The listing builds one solid part. Answer for the finished solid, in the listing's coordinates (mm). Coordinates: 2 decimals unless noted, no trailing zeros. Order: outer loops, then holes, each group sorted by start corner. A loop starts at its lowest first (then second) coordinate and runs counter-clockwise, first axis right, second up. Notation, with made-up numbers: (25, 13.5) -> (83, 13.5) arc R24 ccw to (83, 44.5) -> close; hole circle Ø10 at (-33.75, 76.5). An arc over 180 degrees is marked (long way). One line per question, with ' | ' between items.
from build123d import *

# Parameters (mm, degrees)
BASE_DEPTH                = 3
ESQUISSE3_R               = 2
ESQUISSE3_W               = 65
ESQUISSE3_H               = 30
ENL_V_MAT_EXTRU_1_DEPTH   = 4
CONG_1_R                  = 3
ESQUISSE6_R               = 2
ESQUISSE6_R_2             = 10.5
PER_AGE_POUR_BILLES_DEPTH = 3
PER_AGE_POUR_PROFIL_REACH = 5
ESQUISSE8_R               = 3
ESQUISSE10_R              = 2
ENL_V_MAT_EXTRU_3_DEPTH   = 4
ESQUISSE12_R              = 1.625
ENL_V_MAT_EXTRU_4_DEPTH   = 4
ESQUISSE13_R              = 1.625
ENL_V_MAT_EXTRU_5_DEPTH   = 4


with BuildPart() as part:
    # Esquisse1 → Base (new body)
    with BuildSketch(Plane.XY):
        Polygon((0, 0), (-150, 0), (-174.748737342, 24.748737342), (-174.748737342, 274.748737342), (-150, 299.497474683), (0, 299.497474683), (24.748737342, 274.748737342), (24.748737342, 24.748737342), align=None)
    extrude(amount=BASE_DEPTH)

    # Esquisse3 → Enlèv. mat.-Extru.1 (cut, through all)
    with BuildSketch(Plane(origin=(0, 0, 0), x_dir=(-1, 0, 0), z_dir=(0, 0, -1))):
        with Locations((40, 45)):
            Circle(ESQUISSE3_R)
        with Locations((110, 45)):
            Circle(ESQUISSE3_R)
        with Locations((110, 254.497474683)):
            Circle(ESQUISSE3_R)
        with Locations((40, 254.497474683)):
            Circle(ESQUISSE3_R)
        Polygon((117, 0), (117, 20), (93, 20), (93, 45.5), (57, 45.5), (57, 20), (33, 20), (33, 0), align=None)
        Polygon((33, 299.497474683), (117, 299.497474683), (117, 279.497474683), (93, 279.497474683), (93, 253.997474683), (57, 253.997474683), (57, 279.497474683), (33, 279.497474683), align=None)
        with Locations((75, 229.497474683)):
            Rectangle(ESQUISSE3_W, ESQUISSE3_H)
        with Locations((75, 70)):
            Rectangle(ESQUISSE3_W, ESQUISSE3_H)
    extrude(amount=-ENL_V_MAT_EXTRU_1_DEPTH, mode=Mode.SUBTRACT)

    # Congé1
    cong_1_edges = [part.edges().sort_by_distance(p)[0] for p in [
        (0, 0, 1.5),
        (-150, 0, 1.5),
        (-174.748737342, 24.748737342, 1.5),
        (-174.748737342, 274.748737342, 1.5),
        (-150, 299.497474683, 1.5),
        (0, 299.497474683, 1.5),
        (24.748737342, 274.748737342, 1.5),
        (24.748737342, 24.748737342, 1.5),
        (-33, 279.497474683, 1.5),
        (-33, 299.497474683, 1.5),
        (-117, 299.497474683, 1.5),
        (-117, 279.497474683, 1.5),
        (-93, 279.497474683, 1.5),
        (-93, 253.997474683, 1.5),
        (-57, 253.997474683, 1.5),
        (-57, 279.497474683, 1.5),
        (-117, 0, 1.5),
        (-33, 0, 1.5),
        (-33, 20, 1.5),
        (-57, 20, 1.5),
        (-57, 45.5, 1.5),
        (-93, 45.5, 1.5),
        (-93, 20, 1.5),
        (-117, 20, 1.5),
    ]]
    fillet(cong_1_edges, radius=CONG_1_R)

    # Esquisse6 → Perçage pour billes (cut)
    with BuildSketch(Plane.XY.offset(3)):
        with Locations((-152, 55)):
            Circle(ESQUISSE6_R)
        with Locations((-152, 85)):
            Circle(ESQUISSE6_R)
        with Locations((-152, 70)):
            Circle(ESQUISSE6_R_2)
        with Locations((-5.251262658, 40)):
            Circle(ESQUISSE6_R_2)
        with Locations((-20.251262658, 40)):
            Circle(ESQUISSE6_R)
        with Locations((9.748737342, 40)):
            Circle(ESQUISSE6_R)
    per_age_pour_billes = extrude(amount=-PER_AGE_POUR_BILLES_DEPTH, mode=Mode.SUBTRACT)

    # Esquisse8 → Perçage pour profilé (cut, up to next)
    with BuildSketch(Plane.XY.offset(3), mode=Mode.PRIVATE) as per_age_pour_profil_sk1:
        with Locations((-133, 16)):
            Circle(ESQUISSE8_R)
    per_age_pour_profil_tool1 = extrude(per_age_pour_profil_sk1.sketch, amount=-PER_AGE_POUR_PROFIL_REACH, mode=Mode.PRIVATE) & part.part
    add(per_age_pour_profil_tool1.solids().sort_by_distance((-133, 16, 3))[0], mode=Mode.SUBTRACT)
    # Esquisse8 → Perçage pour profilé (cut, up to next)
    with BuildSketch(Plane.XY.offset(3), mode=Mode.PRIVATE) as per_age_pour_profil_sk2:
        with Locations((-133, 283.497474683)):
            Circle(ESQUISSE8_R)
    per_age_pour_profil_tool2 = extrude(per_age_pour_profil_sk2.sketch, amount=-PER_AGE_POUR_PROFIL_REACH, mode=Mode.PRIVATE) & part.part
    add(per_age_pour_profil_tool2.solids().sort_by_distance((-133, 283.497475, 3))[0], mode=Mode.SUBTRACT)
    # Esquisse8 → Perçage pour profilé (cut, up to next)
    with BuildSketch(Plane.XY.offset(3), mode=Mode.PRIVATE) as per_age_pour_profil_sk3:
        with Locations((-17, 283.497474683)):
            Circle(ESQUISSE8_R)
    per_age_pour_profil_tool3 = extrude(per_age_pour_profil_sk3.sketch, amount=-PER_AGE_POUR_PROFIL_REACH, mode=Mode.PRIVATE) & part.part
    add(per_age_pour_profil_tool3.solids().sort_by_distance((-17, 283.497475, 3))[0], mode=Mode.SUBTRACT)
    # Esquisse8 → Perçage pour profilé (cut, up to next)
    with BuildSketch(Plane.XY.offset(3), mode=Mode.PRIVATE) as per_age_pour_profil_sk4:
        with Locations((-17, 16)):
            Circle(ESQUISSE8_R)
    per_age_pour_profil_tool4 = extrude(per_age_pour_profil_sk4.sketch, amount=-PER_AGE_POUR_PROFIL_REACH, mode=Mode.PRIVATE) & part.part
    add(per_age_pour_profil_tool4.solids().sort_by_distance((-17, 16, 3))[0], mode=Mode.SUBTRACT)

    # Esquisse10 → Enlèv. mat.-Extru.3 (cut, through all)
    with BuildSketch(Plane.XY.offset(3)):
        with Locations((-108, 204.497474683)):
            Circle(ESQUISSE10_R)
        with Locations((-108, 177.997474683)):
            Circle(ESQUISSE10_R)
        with Locations((-42, 177.997474683)):
            Circle(ESQUISSE10_R)
        with Locations((-42, 204.497474683)):
            Circle(ESQUISSE10_R)
        with Locations((-42, 121.5)):
            Circle(ESQUISSE10_R)
        with Locations((-42, 95)):
            Circle(ESQUISSE10_R)
        with Locations((-108, 121.5)):
            Circle(ESQUISSE10_R)
        with Locations((-108, 95)):
            Circle(ESQUISSE10_R)
    extrude(amount=-ENL_V_MAT_EXTRU_3_DEPTH, mode=Mode.SUBTRACT)

    # Symétrie2: Perçage pour billes across plane
    add(per_age_pour_billes.mirror(Plane.ZX.offset(149.748737342)), mode=Mode.SUBTRACT)

    # Esquisse12 → Enlèv. mat.-Extru.4 (cut, through all)
    with BuildSketch(Plane(origin=(0, 0, 0), x_dir=(-1, 0, 0), z_dir=(0, 0, -1))):
        with Locations((-9.748737342, 72.748737342)):
            Circle(ESQUISSE12_R)
        with Locations((-9.748737342, 149.748737342)):
            Circle(ESQUISSE12_R)
        with Locations((-9.748737342, 226.748737342)):
            Circle(ESQUISSE12_R)
        with Locations((18.251262658, 226.748737342)):
            Circle(ESQUISSE12_R)
        with Locations((18.251262658, 149.748737342)):
            Circle(ESQUISSE12_R)
        with Locations((18.251262658, 72.748737342)):
            Circle(ESQUISSE12_R)
    extrude(amount=-ENL_V_MAT_EXTRU_4_DEPTH, mode=Mode.SUBTRACT)

    # Esquisse13 → Enlèv. mat.-Extru.5 (cut, through all)
    with BuildSketch(Plane(origin=(0, 0, 0), x_dir=(-1, 0, 0), z_dir=(0, 0, -1))):
        with Locations((28.501262658, 122.748737342)):
            Circle(ESQUISSE13_R)
        with Locations((28.501262658, 176.748737342)):
            Circle(ESQUISSE13_R)
        with Locations((168.498737342, 119.748737342)):
            Circle(ESQUISSE13_R)
        with Locations((168.498737342, 179.748737342)):
            Circle(ESQUISSE13_R)
    extrude(amount=-ENL_V_MAT_EXTRU_5_DEPTH, mode=Mode.SUBTRACT)


solid = part.part
Item 1: Section B-B, the plane z = 1.8 is taken. Count the separate pieces of the cut face and the enclosed holes in it, plus the area to 3 significant figures.
Computed values:
separate pieces: 1 | enclosed holes: 40 | area: 47,600 mm^2
Item 2: Section A-A, the plane x = -133 is taken. Give the vertices of the cut face in (y, z).
Computed values:
outline: (0, 0) -> (13, 0) -> (13, 3) -> (0, 3) -> close; (19, 0) -> (280.5, 0) -> (280.5, 3) -> (19, 3) -> close; (286.5, 0) -> (299.5, 0) -> (299.5, 3) -> (286.5, 3) -> close
Item 3: Each of these flat-tipped pins is pushed along its axis until it touches: pin 1 Ø5 at (x, y) = (-133, 283.5) entering from +Z; pin 2 Ø5 at (x, y) = (-168.5, 119.75) entering from +Z; pin 3 Ø0.9 at (y, z) = (11, 2) entering from +X; pin 4 Ø1.5 at (x, z) = (-71, 1) entering from +Y. Where does it stop, or does it pass through?
Computed values:
pin 1: passes through | pin 2: stops at z = 3 | pin 3: stops at x = 11.45 | pin 4: stops at y = 254
Item 4: Determine the mould class of faces 1 (the face through (-131.616, 280.836, 1.521)), 2 (the face through (-74, 152, 0)), 3 (the face through (-162.5, 287, 1.5)), 4 (the face through (12.2, 287.3, 1.5)) for opening direction X: pulls with the +X half, pulls with the -X half, needs draft (parallel to the pull), parting line crosses it, or undercut.
Computed values:
face 1: undercut | face 2: needs draft | face 3: pulls with the -X half | face 4: pulls with the +X half
Item 5: Find the intervals of material crossed by L1, parallel to Y at x = -76.5, z = 1.1; L2, parallel to X at y = 95.5, z = 0.15; L3, parallel to Y at x = -44.5, z = 1.5, in increasing order.
Computed values:
L1: y = 45.5 to 55, 85 to 214.5, 244.5 to 254 | L2: x = -174.75 to -109.94, -106.06 to -43.94, -40.06 to 24.75 | L3: y = 20 to 55, 85 to 214.5, 244.5 to 279.5
